Geometry check sheet. Reference: drawing and pictorial views, mm from the part's lowest x, y, z. Coordinates: 2 decimals unless noted, no trailing zeros. Loops run counter-clockwise (first coordinate to the right, second up) from the corner with the lowest first, then second, coordinate; pieces in that order, holes last. Notation, with made-up numbers: (80.25, 82.5) -> (139.25, 82.5) arc R23 cw to (139.25, 121.5) -> close; hole circle Ø9 at (39.5, -0.75). An arc over 180 degrees is marked (long way). Use one line per item in the form item = value.
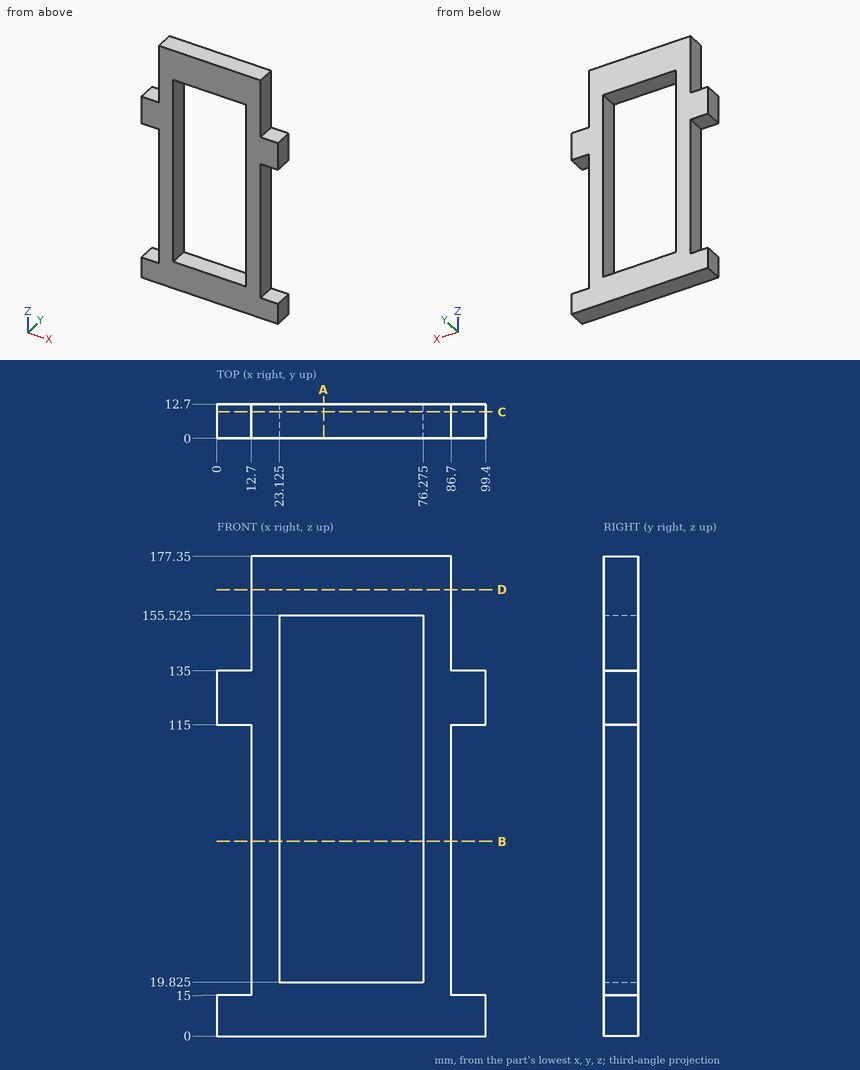
(1) Scan lines: line 1 along X through (y, z) = (10.5, 83.5) (3 decimals); line 2 along Z through (x, y) = (35.5, 12) (3 decimals); line 3 along X through (y, z) = (2.25, 134.5) (3 decimals). Record each from-to range of solid material in increasing order.
Established:
line_1 = 12.7 to 23.125, 76.275 to 86.7
line_2 = 0 to 19.825, 155.525 to 177.35
line_3 = 0 to 23.125, 76.275 to 99.4
(2) Section check B-B, the plane z = 72. Record the boundary of the cut face in (x, y) (3 decimals).
Established:
outline = (12.7, 0) -> (23.125, 0) -> (23.125, 12.7) -> (12.7, 12.7) -> close; (76.275, 0) -> (86.7, 0) -> (86.7, 12.7) -> (76.275, 12.7) -> close
(3) Section check C-C, the plane y = 9.75. Record the boundary of the cut face in (x, z) (3 decimals).
Established:
outline = (0, 0) -> (99.4, 0) -> (99.4, 15) -> (86.7, 15) -> (86.7, 115) -> (99.4, 115) -> (99.4, 135) -> (86.7, 135) -> (86.7, 177.35) -> (12.7, 177.35) -> (12.7, 135) -> (0, 135) -> (0, 115) -> (12.7, 115) -> (12.7, 15) -> (0, 15) -> close; hole (23.125, 19.825) -> (76.275, 19.825) -> (76.275, 155.525) -> (23.125, 155.525) -> close
(4) Section check D-D, the plane z = 165. Record the boundary of the cut face in (x, y).
Established:
outline = (12.7, 0) -> (86.7, 0) -> (86.7, 12.7) -> (12.7, 12.7) -> close
(5) Go/stop test with flat-tipped pins: P1, Ø6.5, axis at y = 8, z = 146.5, coming from the -X side; P2, Ø5, axis at y = 4.5, z = 51.5, coming from the +X side; P3, Ø4, axis at x = 95, y = 4.5, coming from the +Z side. Record where each tip stops, or that it passes through.
Established:
P1 = 12.7
P2 = 86.7
P3 = 135
(6) Section check A-A, the plane x = 39.5. Record the boundary of the cut face in (y, z) (3 decimals).
Established:
outline = (0, 0) -> (12.7, 0) -> (12.7, 19.825) -> (0, 19.825) -> close; (0, 155.525) -> (12.7, 155.525) -> (12.7, 177.35) -> (0, 177.35) -> close
